The drawing under review shows one solid part. Ordinate dimensions are in mm from its lowest x, y, z. A direction names the side the tool comes from. Give positions to 0.01 mm unless a question says otherwise; leave off trailing zeros. Loops run counter-clockwise (first coordinate to the right, second up) from the corner with the lowest first, then second, coordinate; pieces in that order, holes last. Notation, with made-up numbers: (79, 42) - (88, 42) arc R30 ccw to (88, 65) - close; hole circle Ø3 at (86.25, 33). An arc over 180 degrees is marked (long way). Write each question's results on one line, items separated by ' | '.
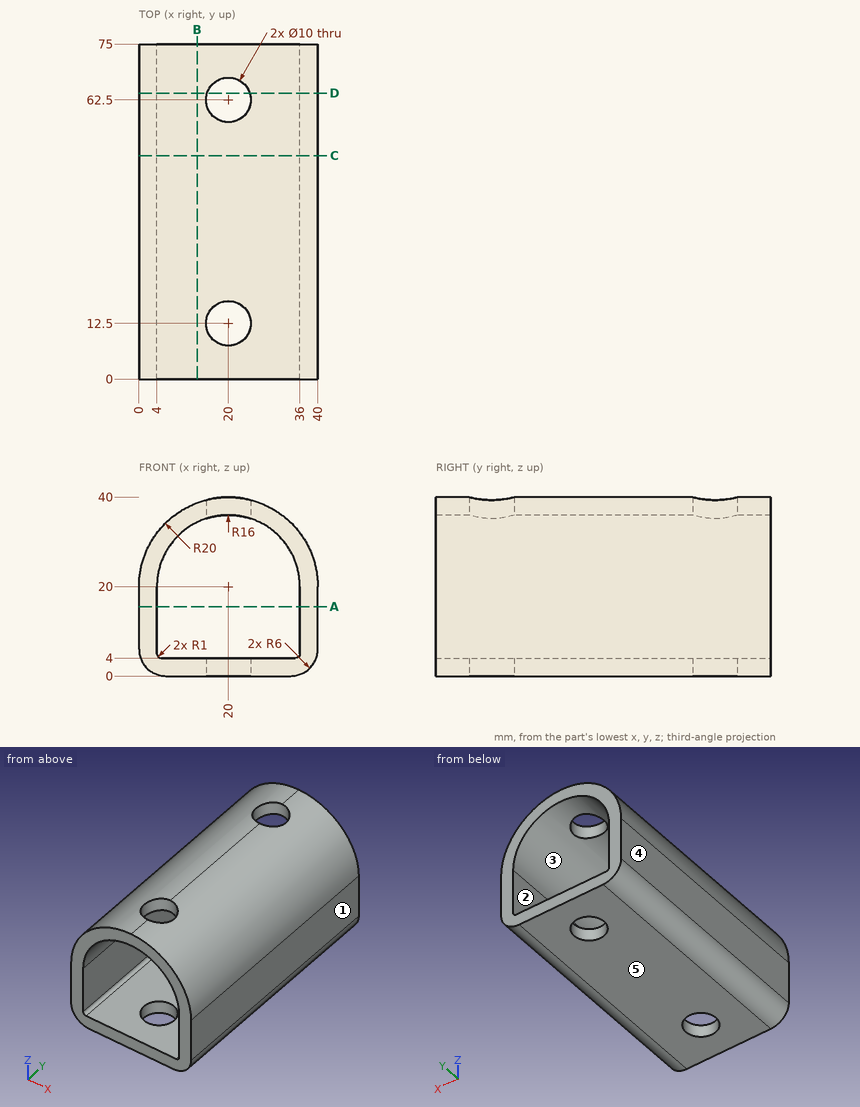
(1) Tool access review of the marked faces 1 and 2: name each direction out of +Z, -Z, +X, -X, +Y, -Y from which nothing blocks a thin tool from reaching the whole face with its end or side.
Answers below:
face 1: +Z, -Z, +X, +Y, -Y | face 2: +Y, -Y
(2) Draft analysis for pull direction Z (two halves, no side actions). For the marked faces 3, 4 and 5, state which applies: pulls with the +Z half, pulls with the -Z half, needs draft (parallel to the pull), parting line crosses it, or undercut.
Answers below:
face 3: undercut | face 4: needs draft | face 5: pulls with the -Z half
(3) Take a section at A-A on z = 15.5. Give the boundary of the cut face in (x, y), plus the area to 3 significant figures.
Answers below:
outline: (0, 0) - (4, 0) - (4, 75) - (0, 75) - close; (36, 0) - (40, 0) - (40, 75) - (36, 75) - close | area: 600 mm2
(4) Take a section at D-D on y = 64. Give the boundary of the cut face in (x, z), plus the area to 3 significant figures.
Answers below:
outline: (0, 6) arc R6 ccw to (6, 0) - (15.23, 0) - (15.23, 4) - (5, 4) arc R1 cw to (4, 5) - (4, 20) arc R16 cw to (15.23, 35.27) - (15.23, 39.42) arc R20 ccw to (0, 20) - close; (24.77, 0) - (34, 0) arc R6 ccw to (40, 6) - (40, 20) arc R20 ccw to (24.77, 39.42) - (24.77, 35.27) arc R16 cw to (36, 20) - (36, 5) arc R1 cw to (35, 4) - (24.77, 4) - close | area: 422 mm2
(5) Wall thickness on line 1 along Y through (x, z) = (20, 2); line 2 along X through (y, z) = (50.5, 7.5); line 3 along X through (y, z) = (62, 2): over which ranges is each line inside the solid? List them lowest first. Write a range as from..to.
Answers below:
line 1: 0..7.5, 17.5..57.5, 67.5..75 | line 2: 0..4, 36..40 | line 3: 1.53..15.03, 24.97..38.47
(6) Take a section at B-B on x = 13. Give the boundary of the cut face in (y, z) (1 decimal), plus the area to 3 significant figures.
Answers below:
outline: (0, 0) - (75, 0) - (75, 4) - (0, 4) - close; (0, 34.4) - (75, 34.4) - (75, 38.7) - (0, 38.7) - close | area: 626 mm2
(7) Take a section at C-C on y = 50. Give the boundary of the cut face in (x, z).
Answers below:
outline: (0, 6) arc R6 ccw to (6, 0) - (34, 0) arc R6 ccw to (40, 6) - (40, 20) arc R20 ccw to (0, 20) - close; hole (4, 5) arc R1 ccw to (5, 4) - (35, 4) arc R1 ccw to (36, 5) - (36, 20) arc R16 ccw to (4, 20) - close
(8) Insertion check: P1, Ø9, axis at x = 20, y = 62.5, coming from the -Z side; P2, Ø1.5, axis at x = 15, y = 29.5, coming from the +Z side; P3, Ø12, axis at y = 43.5, z = 27, coming from the -X side (3 decimals); P4, Ø5, axis at x = 28, y = 45.5, coming from the +Z side. Each pin has a flat end and moves straight along its axis. Give the tip position at first contact, or say it passes through.
Answers below:
P1: through | P2: z = 39.54 | P3: x = 0.025 | P4: z = 39.23
